from build123d import *

# Parameters (mm, degrees)
F1_DEPTH = 84.64962
F1_TAPER = -9
F2_T     = -2.54


with BuildPart() as f1:
    # F0 (on Top) → F1 (new body)
    with BuildSketch(Plane.XY):
        Polygon((32.902453822, -18.9962405711), (0, 37.9924811423), (-32.902453822, -18.9962405711), align=None)
    extrude(amount=F1_DEPTH, taper=F1_TAPER)

    # F2
    f2_openings = [f1.faces().sort_by_distance(p)[0] for p in [
        (22.761478, 13.141345, 46.004837),
    ]]
    offset(amount=F2_T, openings=f2_openings)


solid = f1.part
Could you check a few things on this model? Use its own coordinates, in mm. Round coordinates to 2 decimals unless told otherwise and drop trailing zeros. Use a Markdown table: item, result.
Q1. Thinking about a two-plate mould opening in Z: for faces 1 (the flat face through (-5, -4, 84.65)), 2 (the flat face through (-1, -1, 2.54)), 3 (the flat face through (-3, -2, 0)), which applies, released by +Z, released by -Z, zero draft, split by the parting line, or undercut?
Output values:
| item | result |
|---|---|
| face 1 | released by +Z |
| face 2 | undercut |
| face 3 | released by -Z |
Q2. For pin 1 (2 mm diameter, centred on y = 29.5, z = 70.5, fed in from +X); pin 2 (3 mm diameter, centred on y = 35, z = 48.5, fed in from -X); pin 3 (2 mm diameter, centred on y = 47, z = 29.5, fed in from -X), each with a flat end and sliding along its axis, tell me the tip position at first contact or that it passes through.
Output values:
| item | result |
|---|---|
| pin 1 | x = -14.22 |
| pin 2 | x = -11.51 |
| pin 3 | x = -0.8 |
Q3. Please list where these lines run through material, in increasing order: L1, parallel to Z at x = -4, y = 19.5; L2, parallel to Y at x = -37, z = 56; L3, parallel to Y at x = -14, z = 62.
Output values:
| item | result |
|---|---|
| L1 | 0 to 2.54, 82.11 to 84.65 |
| L2 | -27.87 to -25.29, -13.5 to -8.35 |
| L3 | -28.82 to -26.24, 28.24 to 33.38 |
